Part model, mm, in its own coordinate system. Round coordinates to 2 decimals unless told otherwise and drop trailing zeros. Write each loop counter-clockwise with the first axis right and the second up, starting at its lowest first coordinate (ties: lowest second). Pieces come first, ordered by that corner, then holes. Notation, with made-up numbers: (37, 9) -> (78, 9) arc R20 ccw to (78, 42) -> close; hole circle Ø6 at (47, 4). An arc over 180 degrees is marked (long way). Use CSV: the item, a comma, the result in double quotes. Start each with the question number.
(1) Saw through at A-A (z = 12.5). Count the separate pieces of the cut face and the enclosed holes in it, plus the area to 3 significant figures.
(2) Saw through at B-B (x = -7.5). Give the cut face in (y, z).
(3) Drop flat-ended pins along their axis: pin 1 (4 mm diameter, centred on y = 5.5, z = 23, fed in from -X); pin 2 (1.5 mm diameter, centred on y = 10.5, z = 14.5, fed in from +X). Give the stop position or say it passes through.
(4) Probe line 1 (X direction, y = -8, z = 22.25); line 2 (X direction, y = -2.5, z = 20.25); line 3 (X direction, y = 5.25, z = 17). List the from-to ranges inside material, lowest first. Write a range as [from, to].
(5) Two-plate mould, pull along X, no slides. Class faces 1 (the cylindrical face through (12.07, 12, 12.82)), 2 (the flat face through (3, -9, 12)), 3 (the flat face through (-4, 8.5, 12)): released by +X, released by -X, zero draft, split by the parting line, or undercut.
(6) Saw through at C-C (x = -15). Give the cut face in (y, z), plus the area to 3 significant figures.
```python
from build123d import *

# Parameters (mm, degrees)
BOSS_EXTRU_5_DEPTH = 25
ESQUISSE7_R        = 8
ESQUISSE7_R_2      = 7.5
BOSS_EXTRU_7_DEPTH = 5
BOSS_EXTRU_6_DEPTH = 1


# Read off the part's stored shape, not the designer's step: Boss.-Extru.5
with BuildPart() as part:
    # Boss.-Extru.5 outline → Boss.-Extru.5 (new body)
    # profile 1 of 2: a face of its own
    with BuildSketch(Plane.XY):
        with BuildLine():
            Line((-8.5, -13.5), (8.5, -13.5))
            ThreePointArc((8.5, -13.5), (12.035533906, -12.035533906), (13.5, -8.5))
            Line((13.5, -8.5), (13.5, 8.5))
            ThreePointArc((13.5, 8.5), (12.035533906, 12.035533906), (8.5, 13.5))
            Line((8.5, 13.5), (-8.5, 13.5))
            ThreePointArc((-8.5, 13.5), (-12.035533906, 12.035533906), (-13.5, 8.5))
            Line((-13.5, 8.5), (-13.5, -8.5))
            ThreePointArc((-13.5, -8.5), (-12.035533906, -12.035533906), (-8.5, -13.5))
        make_face()
        with BuildLine():
            Line((-10, 3.5), (-10, 8.5))
            ThreePointArc((-10, 8.5), (-9.560660172, 9.560660172), (-8.5, 10))
            Line((-8.5, 10), (-3.5, 10))
            Line((-3.5, 10), (-3.5, 9.5))
            Line((-3.5, 9.5), (-3, 9.5))
            Line((-3, 9.5), (-3, 8.5))
            Line((-3, 8.5), (-6, 8.5))
            Line((-6, 8.5), (-6, 7.060660172))
            Line((-6, 7.060660172), (-3.439339828, 4.5))
            Line((-3.439339828, 4.5), (-0.866025404, 4.5))
            Line((-0.866025404, 4.5), (0, 4))
            Line((0, 4), (0.866025404, 4.5))
            Line((0.866025404, 4.5), (3.439339828, 4.5))
            Line((3.439339828, 4.5), (6, 7.060660172))
            Line((6, 7.060660172), (6, 8.5))
            Line((6, 8.5), (3, 8.5))
            Line((3, 8.5), (3, 9.5))
            Line((3, 9.5), (3.5, 9.5))
            Line((3.5, 9.5), (3.5, 10))
            Line((3.5, 10), (8.5, 10))
            ThreePointArc((8.5, 10), (9.560660172, 9.560660172), (10, 8.5))
            Line((10, 8.5), (10, 3.5))
            Line((10, 3.5), (9.5, 3.5))
            Line((9.5, 3.5), (9.5, 3))
            Line((9.5, 3), (8.5, 3))
            Line((8.5, 3), (8.5, 6))
            Line((8.5, 6), (7.060660172, 6))
            Line((7.060660172, 6), (4.5, 3.439339828))
            Line((4.5, 3.439339828), (4.5, 0.866025404))
            Line((4.5, 0.866025404), (4, 0))
            Line((4, 0), (4.5, -0.866025404))
            Line((4.5, -0.866025404), (4.5, -3.439339828))
            Line((4.5, -3.439339828), (7.060660172, -6))
            Line((7.060660172, -6), (8.5, -6))
            Line((8.5, -6), (8.5, -3))
            Line((8.5, -3), (9.5, -3))
            Line((9.5, -3), (9.5, -3.5))
            Line((9.5, -3.5), (10, -3.5))
            Line((10, -3.5), (10, -8.5))
            ThreePointArc((10, -8.5), (9.560660172, -9.560660172), (8.5, -10))
            Line((8.5, -10), (3.5, -10))
            Line((3.5, -10), (3.5, -9.5))
            Line((3.5, -9.5), (3, -9.5))
            Line((3, -9.5), (3, -8.5))
            Line((3, -8.5), (6, -8.5))
            Line((6, -8.5), (6, -7.060660172))
            Line((6, -7.060660172), (3.439339828, -4.5))
            Line((3.439339828, -4.5), (0.866025404, -4.5))
            Line((0.866025404, -4.5), (0, -4))
            Line((0, -4), (-0.866025404, -4.5))
            Line((-0.866025404, -4.5), (-3.439339828, -4.5))
            Line((-3.439339828, -4.5), (-6, -7.060660172))
            Line((-6, -7.060660172), (-6, -8.5))
            Line((-6, -8.5), (-3, -8.5))
            Line((-3, -8.5), (-3, -9.5))
            Line((-3, -9.5), (-3.5, -9.5))
            Line((-3.5, -9.5), (-3.5, -10))
            Line((-3.5, -10), (-8.5, -10))
            ThreePointArc((-8.5, -10), (-9.560660172, -9.560660172), (-10, -8.5))
            Line((-10, -8.5), (-10, -3.5))
            Line((-10, -3.5), (-9.5, -3.5))
            Line((-9.5, -3.5), (-9.5, -3))
            Line((-9.5, -3), (-8.5, -3))
            Line((-8.5, -3), (-8.5, -6))
            Line((-8.5, -6), (-7.060660172, -6))
            Line((-7.060660172, -6), (-4.5, -3.439339828))
            Line((-4.5, -3.439339828), (-4.5, -0.866025404))
            Line((-4.5, -0.866025404), (-4, 0))
            Line((-4, 0), (-4.5, 0.866025404))
            Line((-4.5, 0.866025404), (-4.5, 3.439339828))
            Line((-4.5, 3.439339828), (-7.060660172, 6))
            Line((-7.060660172, 6), (-8.5, 6))
            Line((-8.5, 6), (-8.5, 3))
            Line((-8.5, 3), (-9.5, 3))
            Line((-9.5, 3), (-9.5, 3.5))
            Line((-9.5, 3.5), (-10, 3.5))
        make_face(mode=Mode.SUBTRACT)
    # profile 2 of 2: a face of its own
    with BuildSketch(Plane.XY):
        with BuildLine():
            Line((1.949592103, 3.000876196), (1.276279893, 2.435900169))
            ThreePointArc((1.276279893, 2.435900169), (0.001756003, 2.749999439), (-1.273167982, 2.43752811))
            Line((-1.273167982, 2.43752811), (-1.947287092, 3.003181207))
            Line((-1.947287092, 3.003181207), (-3.000876196, 1.949592103))
            Line((-3.000876196, 1.949592103), (-2.435900169, 1.276279893))
            ThreePointArc((-2.435900169, 1.276279893), (-2.749999439, 0.001756003), (-2.43752811, -1.273167982))
            Line((-2.43752811, -1.273167982), (-3.003181207, -1.947287092))
            Line((-3.003181207, -1.947287092), (-1.949592103, -3.000876196))
            Line((-1.949592103, -3.000876196), (-1.276279893, -2.435900169))
            ThreePointArc((-1.276279893, -2.435900169), (-0.001756003, -2.749999439), (1.273167982, -2.43752811))
            Line((1.273167982, -2.43752811), (1.947287092, -3.003181207))
            Line((1.947287092, -3.003181207), (3.000876196, -1.949592103))
            Line((3.000876196, -1.949592103), (2.435900169, -1.276279893))
            ThreePointArc((2.435900169, -1.276279893), (2.749999439, -0.001756003), (2.43752811, 1.273167982))
            Line((2.43752811, 1.273167982), (3.003181207, 1.947287092))
            Line((3.003181207, 1.947287092), (1.949592103, 3.000876196))
        make_face()
    extrude(amount=BOSS_EXTRU_5_DEPTH)

    # Esquisse7 → Boss.-Extru.7 (add)
    with BuildSketch(Plane.ZY.offset(13.5)):
        with Locations(Location((12.5, 0, 0), (0, 0, 180))):
            Circle(ESQUISSE7_R)
        with Locations((12.5, 0)):
            Circle(ESQUISSE7_R_2, mode=Mode.SUBTRACT)
    extrude(amount=BOSS_EXTRU_7_DEPTH)

    # Esquisse6 → Boss.-Extru.6 (add)
    with BuildSketch(Plane.XY.offset(25)):
        with BuildLine():
            Line((-13.5, 8.5), (-13.5, -8.5))
            ThreePointArc((-13.5, -8.5), (-12.035533906, -12.035533906), (-8.5, -13.5))
            Line((-8.5, -13.5), (8.5, -13.5))
            ThreePointArc((8.5, -13.5), (12.035533906, -12.035533906), (13.5, -8.5))
            Line((13.5, -8.5), (13.5, 8.5))
            ThreePointArc((13.5, 8.5), (12.035533906, 12.035533906), (8.5, 13.5))
            Line((8.5, 13.5), (-8.5, 13.5))
            ThreePointArc((-8.5, 13.5), (-12.035533906, 12.035533906), (-13.5, 8.5))
        make_face()
    extrude(amount=BOSS_EXTRU_6_DEPTH)


solid = part.part
```
Answers:
1,separate pieces,"2"
1,enclosed holes,"1"
1,area,"549 mm²"
2,outline,"(-13.5, 0) -> (-10, 0) -> (-10, 25) -> (-6, 25) -> (-6, 0) -> (6, 0) -> (6, 25) -> (10, 25) -> (10, 0) -> (13.5, 0) -> (13.5, 26) -> (-13.5, 26) -> close"
3,pin 1,"stops at x = -13.5"
3,pin 2,"stops at x = 13.34"
4,line 1,"x = [-13.5, -10], [-6, 6], [10, 13.5]"
4,line 2,"x = [-13.5, -4.5], [-2.45, -1.35], [-1.15, 1.15], [1.35, 2.45], [4.5, 13.5]"
4,line 3,"x = [-13.5, -10], [-8.5, -6.31], [-4.19, 4.19], [6.31, 8.5], [10, 13.5]"
5,face 1,"released by +X"
5,face 2,"undercut"
5,face 3,"undercut"
6,outline,"circle Ø16 at (0, 12.5); hole circle Ø15 at (0, 12.5)"
6,area,"24.3 mm²"
